Could you check a few things on this model? Use its own coordinates, in mm. Give positions to 0.01 mm unless a question says otherwise; leave off trailing zeros. Loops run counter-clockwise (first coordinate to the right, second up) from the corner with the lowest first, then second, coordinate; pieces in that order, holes last. Notation, with made-up numbers: (-4.5, 32) -> (26.5, 32) arc R6 ccw to (26.5, 39) -> close; hole circle Ø10 at (89.25, 41.5). An arc over 180 degrees is marked (long way). Put each result on its own line as item: value.
```python
from build123d import *

# Parameters (mm, degrees)
SKETCH1_R               = 88.9
SKETCH1_R_2             = 85.725
BOSS_EXTRUDE1_DEPTH     = 199.39
CUT_EXTRUDE1_REACH      = 237.718
CUT_EXTRUDE1_END_RADIUS = 88.9
SKETCH2_W               = 127
SKETCH2_H               = 360.68
CIRPATTERN1_COUNT       = 3


with BuildPart() as part:
    # Sketch1 → Boss-Extrude1 (new, symmetric)
    with BuildSketch(Plane(origin=(0, 0, 0), x_dir=(1, 0, 0), z_dir=(0, 1, 0))):
        with Locations(Location((0, 0, 0), (0, 0, 270))):
            Circle(SKETCH1_R)
        with Locations(Location((0, 0, 0), (0, 0, 270))):
            Circle(SKETCH1_R_2, mode=Mode.SUBTRACT)
    extrude(amount=BOSS_EXTRUDE1_DEPTH, both=True)

    # Cut-Extrude1: up to this cylinder (the profile starts inside it)
    cut_extrude1_end = Plane(origin=(0, -6.35, 0), z_dir=(0, -1, 0)) * Cylinder(CUT_EXTRUDE1_END_RADIUS, 654.236, mode=Mode.PRIVATE)
    # Sketch2 → Cut-Extrude1 (cut, up to the surface)
    with BuildSketch(Plane.XY, mode=Mode.PRIVATE) as cut_extrude1_sk1:
        with Locations((0, -6.35)):
            Rectangle(SKETCH2_W, SKETCH2_H)
    cut_extrude1_tool1 = extrude(cut_extrude1_sk1.sketch, amount=-CUT_EXTRUDE1_REACH, mode=Mode.PRIVATE) & cut_extrude1_end
    cut_extrude1 = cut_extrude1_tool1.solids().sort_by_distance((0, -6.35, 0))[0]
    add(cut_extrude1, mode=Mode.SUBTRACT)

    # CirPattern1: Cut-Extrude1 ×3 about axis
    cirpattern1_axis = Axis((0, 0, 0), (0, 1, 0))
    for i in range(1, CIRPATTERN1_COUNT):
        add(cut_extrude1.rotate(cirpattern1_axis, i * 360 / CIRPATTERN1_COUNT), mode=Mode.SUBTRACT)


solid = part.part
```
1. If we section it at D-D (x = 28): List the corners of the cut face in (y, z) for me, then the cut area to 3 significant figures.
Recorded:
outline: (-199.39, -84.38) -> (-186.69, -84.38) -> (-186.69, -81.02) -> (-199.39, -81.02) -> close; (-199.39, 81.02) -> (-186.69, 81.02) -> (-186.69, 84.38) -> (-199.39, 84.38) -> close; (173.99, -84.38) -> (199.39, -84.38) -> (199.39, -81.02) -> (173.99, -81.02) -> close; (173.99, 81.02) -> (199.39, 81.02) -> (199.39, 84.38) -> (173.99, 84.38) -> close
area: 255 mm^2
2. If we section it at B-B (z = 0): List the corners of the cut face in (x, y) for me (3 decimals).
Recorded:
outline: (-88.9, -199.39) -> (-85.725, -199.39) -> (-85.725, -186.69) -> (-88.9, -186.69) -> close; (-88.9, 173.99) -> (-85.725, 173.99) -> (-85.725, 199.39) -> (-88.9, 199.39) -> close; (85.725, -199.39) -> (88.9, -199.39) -> (88.9, -186.69) -> (85.725, -186.69) -> close; (85.725, 173.99) -> (88.9, 173.99) -> (88.9, 199.39) -> (85.725, 199.39) -> close
3. I'm going to push flat-ended pins straight in: pin 1 (1 mm diameter, centred on x = -7.5, y = -102, fed in from -Z); pin 2 (6 mm diameter, centred on x = -11.5, y = -4.5, fed in from +Z); pin 3 (1 mm diameter, centred on y = -42.5, z = -30.5, fed in from -X); pin 4 (21 mm diameter, centred on x = -56, z = 53, fed in from -Y). Where does each tip first touch, or does it pass through?
Recorded:
pin 1: stops at z = 85.35
pin 2: stops at z = 88.49
pin 3: stops at x = -83.69
pin 4: stops at y = -199.39
4. Thinking about a two-plate mould opening in X: for faces 1 (the face through (-11.61, 0.93, 88.14)), 2 (the face through (73, 199.39, -47)), 3 (the face through (8.703, 13.839, 85.282)), which applies, pulls with the +X half, pulls with the -X half, needs draft (parallel to the pull), parting line crosses it, or undercut?
Recorded:
face 1: parting line crosses it
face 2: needs draft
face 3: undercut
5. If we section it at A-A (x = 0): List the corners of the cut face in (y, z) for me (3 decimals), then the cut area to 3 significant figures.
Recorded:
outline: (-199.39, -88.9) -> (-186.69, -88.9) -> (-186.69, -85.725) -> (-199.39, -85.725) -> close; (-199.39, 85.725) -> (199.39, 85.725) -> (199.39, 88.9) -> (-199.39, 88.9) -> close; (173.99, -88.9) -> (199.39, -88.9) -> (199.39, -85.725) -> (173.99, -85.725) -> close
area: 1,390 mm^2
6. If we section it at C-C (y = 102.5): List the corners of the cut face in (x, z) for me (3 decimals).
Recorded:
outline: (-85.632, -23.884) arc R88.9 ccw to (-63.5, -62.217) -> (-63.5, -57.589) arc R85.725 cw to (-81.624, -26.198) -> close; (-22.132, 86.101) -> (-18.124, 83.787) arc R85.725 cw to (18.124, 83.787) -> (22.132, 86.101) arc R88.9 ccw to start; (63.5, -62.217) arc R88.9 ccw to (85.632, -23.884) -> (81.624, -26.198) arc R85.725 cw to (63.5, -57.589) -> close
7. I need wall thicknesses on line 1 (Z direction, x = 0, y = 26) (3 decimals); line 2 (X direction, y = -175, z = -35); line 3 (X direction, y = 34, z = -37). Which ranges of each line are inside material? Lowest first, please.
Recorded:
line 1: z = 85.725 to 88.9
line 2: x = -81.72 to -78.25, 78.25 to 81.72
line 3: x = -80.83 to -77.33, 77.33 to 80.83
